The model under review builds one solid part; all positions refer to its coordinate system, in mm. A direction names the side the tool comes from. Coordinates: 2 decimals unless noted, no trailing zeros. Order: outer loops, then holes, each group sorted by start corner. A loop starts at its lowest first (then second) coordinate and runs counter-clockwise, first axis right, second up.
```python
from build123d import *

# Parameters (mm, degrees)
ESBO_O1_W                = 40
ESBO_O1_H                = 40
RESSALTO_EXTRUS_O1_DEPTH = 2.5
FILETE1_R                = 3
FILETE2_R                = 3
ESBO_O2_W                = 31
ESBO_O2_H                = 31
RESSALTO_EXTRUS_O2_DEPTH = 15
FILETE3_R                = 1
FILETE4_R                = 1


with BuildPart() as part:
    # Esboço1 → Ressalto-extrusão1 (new, symmetric)
    with BuildSketch(Plane(origin=(0, 0, 0), x_dir=(1, 0, 0), z_dir=(0, 1, 0))):
        Rectangle(ESBO_O1_W, ESBO_O1_H)
    extrude(amount=RESSALTO_EXTRUS_O1_DEPTH, both=True)

    # Filete1
    filete1_edges = [part.edges().sort_by_distance(p)[0] for p in [
        (-20, 0, -20),
        (20, 0, -20),
        (20, 0, 20),
        (-20, 0, 20),
    ]]
    fillet(filete1_edges, radius=FILETE1_R)

    # Filete2
    filete2_edges = [part.edges().sort_by_distance(p)[0] for p in [
        (-20, 2.5, 0),
        (0, 2.5, -20),
        (0, 2.5, 20),
        (20, 2.5, 0),
        (19.121320344, 2.5, 19.121320344),
        (-19.121320344, 2.5, 19.121320344),
        (19.121320344, 2.5, -19.121320344),
        (-19.121320344, 2.5, -19.121320344),
    ]]
    fillet(filete2_edges, radius=FILETE2_R)

    # Esboço2 → Ressalto-extrusão2 (add)
    with BuildSketch(Plane.XZ.offset(2.5)):
        with BuildLine():
            Line((-18, 17), (-18, -17))
            ThreePointArc((-18, -17), (-17.707106781, -17.707106781), (-17, -18))
            Line((-17, -18), (17, -18))
            ThreePointArc((17, -18), (17.707106781, -17.707106781), (18, -17))
            Line((18, -17), (18, 17))
            ThreePointArc((18, 17), (17.707106781, 17.707106781), (17, 18))
            Line((17, 18), (-17, 18))
            ThreePointArc((-17, 18), (-17.707106781, 17.707106781), (-18, 17))
        make_face()
        Rectangle(ESBO_O2_W, ESBO_O2_H, mode=Mode.SUBTRACT)
    extrude(amount=RESSALTO_EXTRUS_O2_DEPTH)

    # Filete3
    filete3_edges = [part.edges().sort_by_distance(p)[0] for p in [
        (-15.5, -10, 15.5),
        (-15.5, -10, -15.5),
        (15.5, -10, -15.5),
        (15.5, -10, 15.5),
    ]]
    fillet(filete3_edges, radius=FILETE3_R)

    # Filete4
    filete4_edges = [part.edges().sort_by_distance(p)[0] for p in [
        (15.5, -17.5, 0),
        (-15.5, -17.5, 0),
        (0, -17.5, 15.5),
        (15.207106781, -17.5, -15.207106781),
        (-15.207106781, -17.5, -15.207106781),
        (15.207106781, -17.5, 15.207106781),
        (-15.207106781, -17.5, 15.207106781),
        (-17.707106781, -17.5, 17.707106781),
        (-18, -17.5, 0),
        (-17.707106781, -17.5, -17.707106781),
        (0, -17.5, -18),
        (17.707106781, -17.5, -17.707106781),
        (18, -17.5, 0),
        (17.707106781, -17.5, 17.707106781),
        (0, -17.5, 18),
        (0, -17.5, -15.5),
    ]]
    fillet(filete4_edges, radius=FILETE4_R)


solid = part.part
```
(1) Draft analysis for pull direction Z (two halves, no side actions). For faces 6 (the face through (0, -9, -15.5)), 7 (the face through (-19.14, -1.51, -19.1)), 8 (the face through (0, -1, 20)), state which applies: released by +Z, released by -Z, zero draft, split by the parting line, or undercut.
A:
face 6: undercut
face 7: released by -Z
face 8: released by +Z
(2) We need section B-B, the plane x = 13.5. Write out the cut boundary in (y, z), and give its area (3 significant figures).
A:
outline: (-17.5, -17) arc R1 ccw to (-16.5, -18) - (-2.5, -18) - (-2.5, -20) - (-0.5, -20) arc R3 ccw to (2.5, -17) - (2.5, 17) arc R3 ccw to (-0.5, 20) - (-2.5, 20) - (-2.5, 18) - (-16.5, 18) arc R1 ccw to (-17.5, 17) - (-17.5, 16.5) arc R1 ccw to (-16.5, 15.5) - (-2.5, 15.5) - (-2.5, -15.5) - (-16.5, -15.5) arc R1 ccw to (-17.5, -16.5) - close
area: 270 mm2
(3) Wall thickness on probe 1 along X at (y, z) = (-13.25, 4.5); probe 2 along Y at (x, z) = (15, -3): over which ranges is each line inside the solid? List them lowest first.
A:
probe 1: x = -18 to -15.5, 15.5 to 18
probe 2: y = -2.5 to 2.5
(4) We need section C-C, the plane y = -14.25. Write out the cut boundary in (x, z), and give its area (3 significant figures).
A:
outline: (-18, -17) arc R1 ccw to (-17, -18) - (17, -18) arc R1 ccw to (18, -17) - (18, 17) arc R1 ccw to (17, 18) - (-17, 18) arc R1 ccw to (-18, 17) - close; hole (-15.5, -14.5) arc R1 ccw to (-14.5, -15.5) - (14.5, -15.5) arc R1 ccw to (15.5, -14.5) - (15.5, 14.5) arc R1 ccw to (14.5, 15.5) - (-14.5, 15.5) arc R1 ccw to (-15.5, 14.5) - close
area: 335 mm2
(5) We need section D-D, the plane y = 1.25. Write out the cut boundary in (x, z), and give its area (3 significant figures).
A:
outline: (-19.44, -17) arc R2.44 ccw to (-17, -19.44) - (17, -19.44) arc R2.44 ccw to (19.44, -17) - (19.44, 17) arc R2.44 ccw to (17, 19.44) - (-17, 19.44) arc R2.44 ccw to (-19.44, 17) - close
area: 1,510 mm2
(6) For pin 1 Ø4 at (y, z) = (-11.5, -5) entering from -X; pin 2 Ø4 at (y, z) = (-6, 1.5) entering from +X; pin 3 Ø12 at (x, z) = (-8.5, 3.5) entering from -Y, all flat-tipped, find the tip position at first contact; note any pin that passes through.
A:
pin 1: stops at x = -18
pin 2: stops at x = 18
pin 3: stops at y = -2.5
(7) We need section A-A, the plane z = -10.5. Write out the cut boundary in (x, y), and give its area (3 significant figures).
A:
outline: (-20, -2.5) - (-18, -2.5) - (-18, -16.5) arc R1 ccw to (-17, -17.5) - (-16.5, -17.5) arc R1 ccw to (-15.5, -16.5) - (-15.5, -2.5) - (15.5, -2.5) - (15.5, -16.5) arc R1 ccw to (16.5, -17.5) - (17, -17.5) arc R1 ccw to (18, -16.5) - (18, -2.5) - (20, -2.5) - (20, -0.5) arc R3 ccw to (17, 2.5) - (-17, 2.5) arc R3 ccw to (-20, -0.5) - close
area: 270 mm2
(8) Machinability: for faces 1 (the face through (0, -2.5, 0)), 2 (the face through (-17.715, -9.402, -17.699)), 3 (the face through (17.715, -9.402, 17.699)), 4 (the face through (17.699, -9.402, -17.715)), 5 (the face through (-18, -9, 0)), which of the approach directions +Z, -Z, +X, -X, +Y, -Y give a long, thin tool a straight path to every point of the face, cutting with its end or side? Answer none if there is none.
A:
face 1: -Y
face 2: -Z, -X, -Y
face 3: +Z, +X, -Y
face 4: -Z, +X, -Y
face 5: +Z, -Z, -X, -Y
